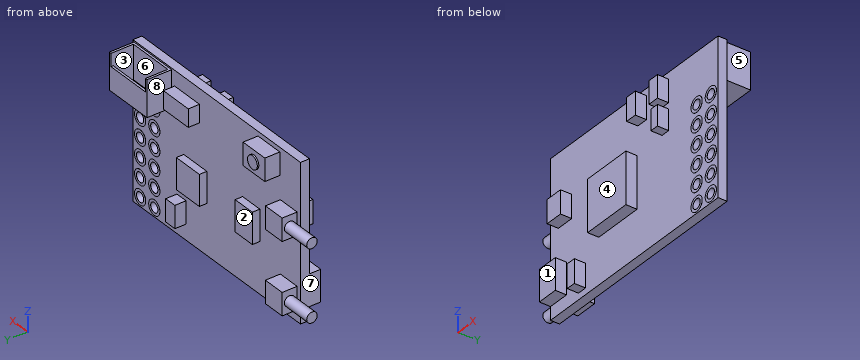
from build123d import *

# Parameters (mm, degrees)
SKETCH1_W            = 30
SKETCH1_H            = 20.65
BOSS_EXTRUDE1_DEPTH  = 1.2
CUT_EXTRUDE1_REACH   = 3.2
SKETCH2_R            = 0.65
SKETCH3_W            = 6.75
SKETCH3_H            = 4.85
BOSS_EXTRUDE2_DEPTH  = 3.3
SKETCH4_W            = 3
SKETCH4_H            = 3
BOSS_EXTRUDE3_DEPTH  = 2
SKETCH5_W            = 3.9
SKETCH5_H            = 3
BOSS_EXTRUDE4_DEPTH  = 2
SKETCH6_R            = 0.875
BOSS_EXTRUDE5_DEPTH  = 0.2
SKETCH7_W            = 6.15
SKETCH7_H            = 1.7
CUT_EXTRUDE2_DEPTH   = 3
SKETCH8_W            = 6.15
SKETCH8_H            = 2.7
CUT_EXTRUDE3_DEPTH   = 2.85
SKETCH9_W            = 4.13358082
SKETCH9_H            = 4.101537558
SKETCH9_W_2          = 3.076153169
SKETCH9_H_2          = 4.13358082
BOSS_EXTRUDE6_DEPTH  = 1
SKETCH10_W           = 1.634206371
SKETCH10_H           = 2.980023382
SKETCH10_W_2         = 4.454013442
SKETCH10_H_2         = 2.371201401
BOSS_EXTRUDE7_DEPTH  = 1.5
SKETCH11_W           = 6.849678862
SKETCH11_H           = 6.849678863
SKETCH11_W_2         = 1.518707079
SKETCH11_H_2         = 3.006420134
SKETCH11_W_3         = 1.5497011
SKETCH11_H_3         = 3.068408178
SKETCH11_W_4         = 1.177772837
SKETCH11_H_4         = 2.758467958
SKETCH11_W_5         = 2.86022906
SKETCH11_H_5         = 4.18419297
SKETCH11_W_6         = 2.386539694
SKETCH11_H_6         = 3.0994022
SKETCH11_W_7         = 1.270754903
SKETCH11_H_7         = 3.161390244
BOSS_EXTRUDE8_DEPTH  = 1.5
SKETCH12_R           = 1
SKETCH12_R_2         = 0.65
BOSS_EXTRUDE9_DEPTH  = 0.01
SKETCH13_R           = 0.7
BOSS_EXTRUDE10_DEPTH = 4


with BuildPart() as part:
    # Sketch1 → Boss-Extrude1 (new body)
    with BuildSketch(Plane(origin=(0, 0, 0), x_dir=(1, 0, 0), z_dir=(0, 1, 0))):
        Rectangle(SKETCH1_W, SKETCH1_H)
    extrude(amount=BOSS_EXTRUDE1_DEPTH)

    # Sketch2 → Cut-Extrude1 (cut, up to next)
    with BuildSketch(Plane(origin=(0, 1.2, 0), x_dir=(1, 0, 0), z_dir=(0, 1, 0)), mode=Mode.PRIVATE) as cut_extrude1_sk1:
        with Locations((13.7, 9.125)):
            Circle(SKETCH2_R)
    cut_extrude1_tool1 = extrude(cut_extrude1_sk1.sketch, amount=-CUT_EXTRUDE1_REACH, mode=Mode.PRIVATE) & part.part
    add(cut_extrude1_tool1.solids().sort_by_distance((13.7, 1.2, -9.125))[0], mode=Mode.SUBTRACT)
    # Sketch2 → Cut-Extrude1 (cut, up to next)
    with BuildSketch(Plane(origin=(0, 1.2, 0), x_dir=(1, 0, 0), z_dir=(0, 1, 0)), mode=Mode.PRIVATE) as cut_extrude1_sk2:
        with Locations((11.16, 9.125)):
            Circle(SKETCH2_R)
    cut_extrude1_tool2 = extrude(cut_extrude1_sk2.sketch, amount=-CUT_EXTRUDE1_REACH, mode=Mode.PRIVATE) & part.part
    add(cut_extrude1_tool2.solids().sort_by_distance((11.16, 1.2, -9.125))[0], mode=Mode.SUBTRACT)
    # Sketch2 → Cut-Extrude1 (cut, up to next)
    with BuildSketch(Plane(origin=(0, 1.2, 0), x_dir=(1, 0, 0), z_dir=(0, 1, 0)), mode=Mode.PRIVATE) as cut_extrude1_sk3:
        with Locations((11.16, 6.585)):
            Circle(SKETCH2_R)
    cut_extrude1_tool3 = extrude(cut_extrude1_sk3.sketch, amount=-CUT_EXTRUDE1_REACH, mode=Mode.PRIVATE) & part.part
    add(cut_extrude1_tool3.solids().sort_by_distance((11.16, 1.2, -6.585))[0], mode=Mode.SUBTRACT)
    # Sketch2 → Cut-Extrude1 (cut, up to next)
    with BuildSketch(Plane(origin=(0, 1.2, 0), x_dir=(1, 0, 0), z_dir=(0, 1, 0)), mode=Mode.PRIVATE) as cut_extrude1_sk4:
        with Locations((11.16, 4.045)):
            Circle(SKETCH2_R)
    cut_extrude1_tool4 = extrude(cut_extrude1_sk4.sketch, amount=-CUT_EXTRUDE1_REACH, mode=Mode.PRIVATE) & part.part
    add(cut_extrude1_tool4.solids().sort_by_distance((11.16, 1.2, -4.045))[0], mode=Mode.SUBTRACT)
    # Sketch2 → Cut-Extrude1 (cut, up to next)
    with BuildSketch(Plane(origin=(0, 1.2, 0), x_dir=(1, 0, 0), z_dir=(0, 1, 0)), mode=Mode.PRIVATE) as cut_extrude1_sk5:
        with Locations((11.16, 1.505)):
            Circle(SKETCH2_R)
    cut_extrude1_tool5 = extrude(cut_extrude1_sk5.sketch, amount=-CUT_EXTRUDE1_REACH, mode=Mode.PRIVATE) & part.part
    add(cut_extrude1_tool5.solids().sort_by_distance((11.16, 1.2, -1.505))[0], mode=Mode.SUBTRACT)
    # Sketch2 → Cut-Extrude1 (cut, up to next)
    with BuildSketch(Plane(origin=(0, 1.2, 0), x_dir=(1, 0, 0), z_dir=(0, 1, 0)), mode=Mode.PRIVATE) as cut_extrude1_sk6:
        with Locations((11.16, -1.035)):
            Circle(SKETCH2_R)
    cut_extrude1_tool6 = extrude(cut_extrude1_sk6.sketch, amount=-CUT_EXTRUDE1_REACH, mode=Mode.PRIVATE) & part.part
    add(cut_extrude1_tool6.solids().sort_by_distance((11.16, 1.2, 1.035))[0], mode=Mode.SUBTRACT)
    # Sketch2 → Cut-Extrude1 (cut, up to next)
    with BuildSketch(Plane(origin=(0, 1.2, 0), x_dir=(1, 0, 0), z_dir=(0, 1, 0)), mode=Mode.PRIVATE) as cut_extrude1_sk7:
        with Locations((11.16, -3.575)):
            Circle(SKETCH2_R)
    cut_extrude1_tool7 = extrude(cut_extrude1_sk7.sketch, amount=-CUT_EXTRUDE1_REACH, mode=Mode.PRIVATE) & part.part
    add(cut_extrude1_tool7.solids().sort_by_distance((11.16, 1.2, 3.575))[0], mode=Mode.SUBTRACT)
    # Sketch2 → Cut-Extrude1 (cut, up to next)
    with BuildSketch(Plane(origin=(0, 1.2, 0), x_dir=(1, 0, 0), z_dir=(0, 1, 0)), mode=Mode.PRIVATE) as cut_extrude1_sk8:
        with Locations((13.7, 6.585)):
            Circle(SKETCH2_R)
    cut_extrude1_tool8 = extrude(cut_extrude1_sk8.sketch, amount=-CUT_EXTRUDE1_REACH, mode=Mode.PRIVATE) & part.part
    add(cut_extrude1_tool8.solids().sort_by_distance((13.7, 1.2, -6.585))[0], mode=Mode.SUBTRACT)
    # Sketch2 → Cut-Extrude1 (cut, up to next)
    with BuildSketch(Plane(origin=(0, 1.2, 0), x_dir=(1, 0, 0), z_dir=(0, 1, 0)), mode=Mode.PRIVATE) as cut_extrude1_sk9:
        with Locations((13.7, 4.045)):
            Circle(SKETCH2_R)
    cut_extrude1_tool9 = extrude(cut_extrude1_sk9.sketch, amount=-CUT_EXTRUDE1_REACH, mode=Mode.PRIVATE) & part.part
    add(cut_extrude1_tool9.solids().sort_by_distance((13.7, 1.2, -4.045))[0], mode=Mode.SUBTRACT)
    # Sketch2 → Cut-Extrude1 (cut, up to next)
    with BuildSketch(Plane(origin=(0, 1.2, 0), x_dir=(1, 0, 0), z_dir=(0, 1, 0)), mode=Mode.PRIVATE) as cut_extrude1_sk10:
        with Locations((13.7, 1.505)):
            Circle(SKETCH2_R)
    cut_extrude1_tool10 = extrude(cut_extrude1_sk10.sketch, amount=-CUT_EXTRUDE1_REACH, mode=Mode.PRIVATE) & part.part
    add(cut_extrude1_tool10.solids().sort_by_distance((13.7, 1.2, -1.505))[0], mode=Mode.SUBTRACT)
    # Sketch2 → Cut-Extrude1 (cut, up to next)
    with BuildSketch(Plane(origin=(0, 1.2, 0), x_dir=(1, 0, 0), z_dir=(0, 1, 0)), mode=Mode.PRIVATE) as cut_extrude1_sk11:
        with Locations((13.7, -1.035)):
            Circle(SKETCH2_R)
    cut_extrude1_tool11 = extrude(cut_extrude1_sk11.sketch, amount=-CUT_EXTRUDE1_REACH, mode=Mode.PRIVATE) & part.part
    add(cut_extrude1_tool11.solids().sort_by_distance((13.7, 1.2, 1.035))[0], mode=Mode.SUBTRACT)
    # Sketch2 → Cut-Extrude1 (cut, up to next)
    with BuildSketch(Plane(origin=(0, 1.2, 0), x_dir=(1, 0, 0), z_dir=(0, 1, 0)), mode=Mode.PRIVATE) as cut_extrude1_sk12:
        with Locations((13.7, -3.575)):
            Circle(SKETCH2_R)
    cut_extrude1_tool12 = extrude(cut_extrude1_sk12.sketch, amount=-CUT_EXTRUDE1_REACH, mode=Mode.PRIVATE) & part.part
    add(cut_extrude1_tool12.solids().sort_by_distance((13.7, 1.2, 3.575))[0], mode=Mode.SUBTRACT)

    # Sketch3 → Boss-Extrude2 (add)
    with BuildSketch(Plane(origin=(0, 1.2, 0), x_dir=(1, 0, 0), z_dir=(0, 1, 0))):
        with Locations((11.425, -7.7)):
            Rectangle(SKETCH3_W, SKETCH3_H)
    extrude(amount=BOSS_EXTRUDE2_DEPTH)

    # Sketch4 → Boss-Extrude3 (add)
    with BuildSketch(Plane(origin=(0, 1.2, 0), x_dir=(1, 0, 0), z_dir=(0, 1, 0))):
        with Locations((-12.9, 7.325)):
            Rectangle(SKETCH4_W, SKETCH4_H)
        with Locations((-12.9, -2.175)):
            Rectangle(SKETCH4_W, SKETCH4_H)
    extrude(amount=BOSS_EXTRUDE3_DEPTH)

    # Sketch5 → Boss-Extrude4 (add)
    with BuildSketch(Plane(origin=(0, 1.2, 0), x_dir=(1, 0, 0), z_dir=(0, 1, 0))):
        with Locations((-9.35, -8.225)):
            Rectangle(SKETCH5_W, SKETCH5_H)
    extrude(amount=BOSS_EXTRUDE4_DEPTH)

    # Sketch6 → Boss-Extrude5 (add)
    with BuildSketch(Plane(origin=(0, 3.2, 0), x_dir=(1, 0, 0), z_dir=(0, 1, 0))):
        with Locations((-9.35, -8.225)):
            Circle(SKETCH6_R)
    extrude(amount=BOSS_EXTRUDE5_DEPTH)

    # Sketch7 → Cut-Extrude2 (cut)
    with BuildSketch(Plane(origin=(0, 4.5, 0), x_dir=(1, 0, 0), z_dir=(0, 1, 0))):
        with Locations((11.425, -9.275)):
            Rectangle(SKETCH7_W, SKETCH7_H)
    extrude(amount=-CUT_EXTRUDE2_DEPTH, mode=Mode.SUBTRACT)

    # Sketch8 → Cut-Extrude3 (cut)
    with BuildSketch(Plane.XY.offset(8.425)):
        with Locations((11.425, 2.85)):
            Rectangle(SKETCH8_W, SKETCH8_H)
    extrude(amount=-CUT_EXTRUDE3_DEPTH, mode=Mode.SUBTRACT)

    # Sketch9 → Boss-Extrude6 (add)
    with BuildSketch(Plane(origin=(0, 1.2, 0), x_dir=(1, 0, 0), z_dir=(0, 1, 0))):
        with Locations((3.82916983, 1.634206371)):
            Rectangle(SKETCH9_W, SKETCH9_H)
        with Locations((-6.1843496, 1.522054953)):
            Rectangle(SKETCH9_W_2, SKETCH9_H_2)
    extrude(amount=BOSS_EXTRUDE6_DEPTH)

    # Sketch10 → Boss-Extrude7 (add)
    with BuildSketch(Plane(origin=(0, 1.2, 0), x_dir=(1, 0, 0), z_dir=(0, 1, 0))):
        with Locations((6.296501018, 6.77714995)):
            Rectangle(SKETCH10_W, SKETCH10_H)
        with Locations((5.30315989, -7.113604202)):
            Rectangle(SKETCH10_W_2, SKETCH10_H_2)
    extrude(amount=BOSS_EXTRUDE7_DEPTH)

    # Sketch11 → Boss-Extrude8 (add)
    with BuildSketch(Plane.XZ):
        with Locations((-2.928935079, -0.803882292)):
            Rectangle(SKETCH11_W, SKETCH11_H)
        with Locations((5.387348503, 7.936431913)):
            Rectangle(SKETCH11_W_2, SKETCH11_H_2)
        with Locations((1.404616675, 7.874443869)):
            Rectangle(SKETCH11_W_3, SKETCH11_H_3)
        with Locations((5.557815623, 4.248143295)):
            Rectangle(SKETCH11_W_4, SKETCH11_H_4)
        with Locations((-13.56988547, -6.475788318)):
            Rectangle(SKETCH11_W_5, SKETCH11_H_5)
        with Locations((-12.403220127, 2.249028876)):
            Rectangle(SKETCH11_W_6, SKETCH11_H_6)
        with Locations((-9.365805971, -7.886016319)):
            Rectangle(SKETCH11_W_7, SKETCH11_H_7)
    extrude(amount=BOSS_EXTRUDE8_DEPTH)

    # Sketch12 → Boss-Extrude9 (add)
    with BuildSketch(Plane(origin=(0, 1.2, 0), x_dir=(1, 0, 0), z_dir=(0, 1, 0))):
        with Locations((11.16, 9.125)):
            Circle(SKETCH12_R)
        with Locations((11.16, 9.125)):
            Circle(SKETCH12_R_2, mode=Mode.SUBTRACT)
        with Locations((13.7, 9.125)):
            Circle(SKETCH12_R)
        with Locations((13.7, 9.125)):
            Circle(SKETCH12_R_2, mode=Mode.SUBTRACT)
        with Locations((13.7, 6.585)):
            Circle(SKETCH12_R)
        with Locations((13.7, 6.585)):
            Circle(SKETCH12_R_2, mode=Mode.SUBTRACT)
        with Locations((11.16, 6.585)):
            Circle(SKETCH12_R)
        with Locations((11.16, 6.585)):
            Circle(SKETCH12_R_2, mode=Mode.SUBTRACT)
        with Locations((11.16, 4.045)):
            Circle(SKETCH12_R)
        with Locations((11.16, 4.045)):
            Circle(SKETCH12_R_2, mode=Mode.SUBTRACT)
        with Locations((13.7, 4.045)):
            Circle(SKETCH12_R)
        with Locations((13.7, 4.045)):
            Circle(SKETCH12_R_2, mode=Mode.SUBTRACT)
        with Locations((13.7, 1.505)):
            Circle(SKETCH12_R)
        with Locations((13.7, 1.505)):
            Circle(SKETCH12_R_2, mode=Mode.SUBTRACT)
        with Locations((11.16, 1.505)):
            Circle(SKETCH12_R)
        with Locations((11.16, 1.505)):
            Circle(SKETCH12_R_2, mode=Mode.SUBTRACT)
        with Locations((11.16, -1.035)):
            Circle(SKETCH12_R)
        with Locations((11.16, -1.035)):
            Circle(SKETCH12_R_2, mode=Mode.SUBTRACT)
        with Locations((11.16, -3.575)):
            Circle(SKETCH12_R)
        with Locations((11.16, -3.575)):
            Circle(SKETCH12_R_2, mode=Mode.SUBTRACT)
        with Locations((13.7, -3.575)):
            Circle(SKETCH12_R)
        with Locations((13.7, -3.575)):
            Circle(SKETCH12_R_2, mode=Mode.SUBTRACT)
        with Locations((13.7, -1.035)):
            Circle(SKETCH12_R)
        with Locations((13.7, -1.035)):
            Circle(SKETCH12_R_2, mode=Mode.SUBTRACT)
    boss_extrude9 = extrude(amount=BOSS_EXTRUDE9_DEPTH)

    # Mirror1: Boss-Extrude9 across plane
    add(boss_extrude9.mirror(Plane.ZX.offset(0.6)))

    # Sketch13 → Boss-Extrude10 (add)
    with BuildSketch(Plane.ZY.offset(14.4)):
        with Locations((-7.325, 2.2)):
            Circle(SKETCH13_R)
        with Locations((2.175, 2.2)):
            Circle(SKETCH13_R)
    extrude(amount=BOSS_EXTRUDE10_DEPTH)


solid = part.part
For this review, take the finished solid that the model builds, in its own axes (mm). Face numbers are marked on the shaded views. A direction names the side the tool comes from. Coordinates: 2 decimals unless noted, no trailing zeros. Loops run counter-clockwise (first coordinate to the right, second up) from the corner with the lowest first, then second, coordinate; pieces in that order, holes last. Notation, with made-up numbers: (85, 21) - (108, 21) arc R32 cw to (108, 57) - close; hole circle Ø7 at (8, -4.5). An arc over 180 degrees is marked (long way). Use a Markdown table: item, result. Add a question column.
Item 1: For line 1 (X direction, y = 2.2, z = 8); line 2 (X direction, y = 0.6, z = -6.5); line 3 (X direction, y = 2.9, z = 9), list the stretches that pass through material, from the lowest coordinate up.
Item 2: Mouldability with a two-part tool opening along Y and no side actions: class the marked faces 1, 2 and 3 as pulls with the +Y half, pulls with the -Y half, needs draft (parallel to the pull), parting line crosses it, or undercut.
Item 3: We need section C-C (x = 11.16). Give the number of separate pieces and of enclosed holes in the cut face, and give its area (3 significant figures).
Item 4: Tool access review of the marked faces 4, 5, 6, 7 and 8: name each direction out of +Z, -Z, +X, -X, +Y, -Y from which nothing blocks a thin tool from reaching the whole face with its end or side.
Item 5: Insertion check: pin 1 Ø2 at (x, z) = (11, -6) entering from -Y; pin 2 Ø3 at (x, y) = (4, 2) entering from -Z (3 decimals); pin 3 Ø2 at (y, z) = (0, -1.5) entering from -X; pin 4 Ø0.8 at (y, z) = (-0.5, 8) entering from +X. Each pin has a flat end and moves straight along its axis. Give the tip position at first contact, or say it passes through.
Item 6: We need section A-A (y = -0.65). Give the boundary of the cut face in (x, z), and give its area (3 significant figures).
Item 7: We need section B-B (x = -2.5). Give the boundary of the cut face in (y, z) (3 decimals).
Item 8: We need section D-D (x = -9.35). Give the boundary of the cut face in (y, z) (3 decimals).
Results list:
| question | item | result |
|---|---|---|
| 1 | line 1 | x = -11.3 to -7.4, 3.08 to 7.53, 8.05 to 8.35, 14.5 to 14.8 |
| 1 | line 2 | x = -15 to 10.52, 11.8 to 13.06, 14.34 to 15 |
| 1 | line 3 | x = -11.3 to -7.4, 8.05 to 8.35, 14.5 to 14.8 |
| 2 | face 1 | pulls with the -Y half |
| 2 | face 2 | pulls with the +Y half |
| 2 | face 3 | undercut |
| 3 | separate pieces | 7 |
| 3 | enclosed holes | 0 |
| 3 | area | 18.7 mm^2 |
| 4 | face 4 | +Z, -Z, +X, -X, -Y |
| 4 | face 5 | +Z, -Z, +X, +Y |
| 4 | face 6 | +Z |
| 4 | face 7 | +Z, -Z, -X, -Y |
| 4 | face 8 | +Z, -Z, +Y |
| 5 | pin 1 | stops at y = -0.01 |
| 5 | pin 2 | stops at z = -10.325 |
| 5 | pin 3 | stops at x = -15 |
| 5 | pin 4 | stops at x = 6.15 |
| 6 | outline | (-15, -8.57) - (-12.14, -8.57) - (-12.14, -4.38) - (-15, -4.38) - close; (-13.6, 0.7) - (-11.21, 0.7) - (-11.21, 3.8) - (-13.6, 3.8) - close; (-10, -9.47) - (-8.73, -9.47) - (-8.73, -6.31) - (-10, -6.31) - close; (-6.35, -4.23) - (0.5, -4.23) - (0.5, 2.62) - (-6.35, 2.62) - close; (0.63, 6.34) - (2.18, 6.34) - (2.18, 9.41) - (0.63, 9.41) - close; (4.63, 6.43) - (6.15, 6.43) - (6.15, 9.44) - (4.63, 9.44) - close; (4.97, 2.87) - (6.15, 2.87) - (6.15, 5.63) - (4.97, 5.63) - close |
| 6 | area | 82.9 mm^2 |
| 7 | outline | (-1.5, -4.229) - (0, -4.229) - (0, -10.325) - (1.2, -10.325) - (1.2, 10.325) - (0, 10.325) - (0, 2.621) - (-1.5, 2.621) - close |
| 8 | outline | (-1.5, -9.467) - (0, -9.467) - (0, -10.325) - (1.2, -10.325) - (1.2, 6.725) - (3.2, 6.725) - (3.2, 7.35) - (3.4, 7.35) - (3.4, 9.1) - (3.2, 9.1) - (3.2, 9.725) - (1.2, 9.725) - (1.2, 10.325) - (0, 10.325) - (0, -6.305) - (-1.5, -6.305) - close |
